Geometry: final body of the model. Coordinates: model frame, mm. A direction names the side the tool comes from. Coordinates: 2 decimals unless noted, no trailing zeros. Loops run counter-clockwise (first coordinate to the right, second up) from the corner with the lowest first, then second, coordinate; pieces in that order, holes last. Notation, with made-up numbers: (-11.75, 28.5) - (6.25, 28.5) arc R20 cw to (6.25, 43.5) - close; hole circle Ø3 at (14, 5). An arc over 180 degrees is marked (long way). Put each result on its own line as item: value. Start each with the question number.
1) Section A-A on x = -14.5. Output: boundary loops of the cut face in (y, z), and give its area (3 significant figures).
2) Reachability of faces 1 (the flat face through (-32, 28, -6)), 2 (the flat face through (-17, 60, -6)) from +Z, -Z, +X, -X, +Y, -Y: full face, straight path, thin tool, end or side. Return the list, or none.
3) Section C-C on z = -9. Output: boundary loops of the cut face in (x, y), and give its area (3 significant figures).
4) Draft query along Z for faces 3 (the flat face through (-22, 0, -14)), 4 (the flat face through (-16, 28, 0)), 5 (the flat face through (-17, 29, -15)). Return one class per face: +Z half, -Z half, draft (parallel to the pull), parting line (faces both ways), or undercut.
5) Contact query for flat-ended pins moving along their axis: pin 1 Ø8 at (x, z) = (-9, -7) entering from -Y; pin 2 Ø3 at (y, z) = (25, -9) entering from +X. Output: stop coordinate, or through.
6) Material intervals for line 1 along Z through (x, y) = (-3, 48); line 2 along X through (y, z) = (34.5, -7.75); line 3 along Y through (x, z) = (-16, -0.5), sorted ascending. Write a range as from..to.
7) Section B-B on y = 5. Output: boundary loops of the cut face in (x, z), and give its area (3 significant figures).
```python
from build123d import *

# Parameters (mm, degrees)
BOSS_EXTRUDE1_DEPTH = 57
SKETCH2_W           = 35
SKETCH2_H           = 18
BOSS_EXTRUDE2_DEPTH = 3
FILLET1_R           = 2


with BuildPart() as part:
    # Sketch1 → Boss-Extrude1 (new body)
    with BuildSketch(Plane(origin=(0, 0, 0), x_dir=(1, 0, 0), z_dir=(0, 1, 0))):
        Polygon((0, 0), (-32, 0), (-32, 12), (0, 12), (0, 15), (-35, 15), (-35, -3), (0, -3), align=None)
    extrude(amount=BOSS_EXTRUDE1_DEPTH)

    # Sketch2 → Boss-Extrude2 (add)
    with BuildSketch(Plane(origin=(0, 57, 0), x_dir=(1, 0, 0), z_dir=(0, 1, 0))):
        with Locations((-17.5, 6)):
            Rectangle(SKETCH2_W, SKETCH2_H)
    extrude(amount=BOSS_EXTRUDE2_DEPTH)

    # Fillet1
    fillet1_edges = [part.edges().sort_by_distance(p)[0] for p in [
        (-35, 30, 3),
        (-35, 30, -15),
        (-35, 60, -6),
        (-17.5, 60, 3),
        (-17.5, 60, -15),
    ]]
    fillet(fillet1_edges, radius=FILLET1_R)


solid = part.part
```
Answer block:
1. outline: (0, -15) - (58, -15) arc R2 ccw to (60, -13) - (60, 1) arc R2 ccw to (58, 3) - (0, 3) - (0, 0) - (57, 0) - (57, -12) - (0, -12) - close
1. area: 394 mm²
2. face 1: +X, -Y
2. face 2: +Z, -Z, +X, -X, +Y
3. outline: (-35, 0) - (-32, 0) - (-32, 57) - (0, 57) - (0, 60) - (-33, 60) arc R2 ccw to (-35, 58) - close
3. area: 275 mm²
4. face 3: draft
4. face 4: undercut
4. face 5: -Z half
5. pin 1: stops at y = 57
5. pin 2: stops at x = -32
6. line 1: z = -15..-12, 0..3
6. line 2: x = -35..-32
6. line 3: y = 57..60
7. outline: (-35, -13) arc R2 ccw to (-33, -15) - (0, -15) - (0, -12) - (-32, -12) - (-32, 0) - (0, 0) - (0, 3) - (-33, 3) arc R2 ccw to (-35, 1) - close
7. area: 244 mm²
